```python
from build123d import *

# Parameters (mm, degrees)
F1_R      = 1
F2_DEPTH  = 2.2
F4_DEPTH  = 0.25
F6_DEPTH  = 2.2
F9_DEPTH  = 30
F11_DEPTH = 6.4
F13_R     = 2
F13_R_2   = 1
F14_DEPTH = 1


# Not quite as in the source:
# - a feature names something its author has since deleted; it is built from what else it names


with BuildPart() as f2:
    # F1 (on Front) → F2 (new body)
    with BuildSketch(Plane.XZ):
        with BuildLine():
            Line((7.35, 2), (7.35, 8.5))
            Line((7.35, 8.5), (0, 8.5))
            ThreePointArc((0, 8.5), (-2.1213203436, 7.6213203436), (-3, 5.5))
            Line((-3, 5.5), (-3, 5))
            ThreePointArc((-3, 5), (-2.8977774789, 4.2235428647), (-2.5980762114, 3.5))
            Line((-2.5980762114, 3.5), (-0.5775284417, 0.0003086038))
            Line((-0.5775284417, 0.0003086038), (0, -1))
            Line((0, -1), (0, 0))
            Line((0, 0), (2, 0))
            Line((2, 0), (7.35, 0))
            Line((7.35, 0), (7.35, 2))
        make_face()
        with Locations((0, 5)):
            Circle(F1_R, mode=Mode.SUBTRACT)
    extrude(amount=-F2_DEPTH)

    # F3 (on Front) → F4 (join)
    with BuildSketch(Plane.XZ):
        Polygon((7.35, 8.5), (4, 8.5), (4, 2), (4, 0), (7.35, 0), (7.35, 2), align=None)
    extrude(amount=F4_DEPTH)

    # F5 (on face) → F6 (join)
    with BuildSketch(Plane.XZ.offset(0.25)):
        with BuildLine():
            ThreePointArc((13.9434358481, 3.491991213), (14.2465762155, 4.2190734812), (14.35, 5))
            Line((14.35, 5), (14.35, 5.5))
            ThreePointArc((14.35, 5.5), (13.4713203436, 7.6213203436), (11.35, 8.5))
            Line((11.35, 8.5), (4, 8.5))
            Line((4, 8.5), (4, 2))
            Line((4, 2), (4, 0))
            Line((4, 0), (7.3888939805, 0))
            Line((7.3888939805, 0), (10.75, -1))
            Line((10.75, -1), (10.75, -2))
            Line((10.75, -2), (13.9434358481, 3.491991213))
        make_face()
        with BuildLine():
            Line((11.35, 3.5), (9.85, 3.5))
            ThreePointArc((9.85, 3.5), (8.35, 5), (9.85, 6.5))
            Line((9.85, 6.5), (11.35, 6.5))
            ThreePointArc((11.35, 6.5), (12.85, 5), (11.35, 3.5))
        make_face(mode=Mode.SUBTRACT)
    extrude(amount=F6_DEPTH)

    # F8 (on offset) → F9 (join)
    with BuildSketch(Plane.XZ.offset(6.45)):
        with BuildLine():
            Line((10.75, -2), (10.75, -1))
            Line((10.75, -1), (10.75, -0.9))
            ThreePointArc((10.75, -0.9), (10.4863961031, -0.2636038969), (9.85, 0))
            Line((9.85, 0), (7.3888939805, 0))
            Line((7.3888939805, 0), (7.3888939805, 0.6))
            ThreePointArc((7.3888939805, 0.6), (7.1252900836, 1.2363961031), (6.4888939805, 1.5))
            Line((6.4888939805, 1.5), (0.9, 1.5))
            ThreePointArc((0.9, 1.5), (0.2636038969, 1.2363961031), (0, 0.6))
            Line((0, 0.6), (0, -1))
            Line((0, -1), (0.5773502692, -2))
            Line((0.5773502692, -2), (2.6773502692, -2))
            Line((2.6773502692, -2), (2.6773502692, -1))
            Line((2.6773502692, -1), (4.6136751346, -1))
            Line((4.6136751346, -1), (4.6136751346, -2))
            Line((4.6136751346, -2), (6.7136751346, -2))
            Line((6.7136751346, -2), (6.7136751346, -1))
            Line((6.7136751346, -1), (8.65, -1))
            Line((8.65, -1), (8.65, -2))
            Line((8.65, -2), (10.75, -2))
        make_face()
    extrude(amount=-F9_DEPTH)

    # F10 (on offset) → F11 (cut)
    with BuildSketch(Plane.XZ.offset(6.45)):
        with BuildLine():
            ThreePointArc((0.9, 1.5), (0.2636038969, 1.2363961031), (0, 0.6))
            Line((0, 0.6), (0, -1))
            Line((0, -1), (0.5773502692, -2))
            Line((0.5773502692, -2), (2.0773502692, -2))
            Line((2.0773502692, -2), (2.0773502692, -0.8))
            Line((2.0773502692, -0.8), (3.6773515204, 1.5))
            Line((3.6773515204, 1.5), (0.9, 1.5))
        make_face()
    extrude(amount=-F11_DEPTH, mode=Mode.SUBTRACT)

    # F12: F2 across plane


with BuildPart() as f2_1:
    add(f2.part)
    add(f2.part.mirror(Plane(origin=(8.5554041441, -6.45, 4.0498921838), x_dir=(1, 0, 0), z_dir=(0, -1, 0))))

    # F13 (on face) → F14 (cut)
    with BuildSketch(Plane.XZ.offset(15.1)):
        with Locations((0, 5)):
            Circle(F13_R)
        with Locations((0, 5)):
            Circle(F13_R_2, mode=Mode.SUBTRACT)
    extrude(amount=-F14_DEPTH, mode=Mode.SUBTRACT)


solid = f2_1.part
```
Design review of the part built by this model. Coordinates are the model's own, in mm. A direction names the side the tool comes from. Round coordinates to 2 decimals unless told otherwise and drop trailing zeros. Write each loop counter-clockwise with the first axis right and the second up, starting at its lowest first coordinate (ties: lowest second). Pieces come first, ordered by that corner, then holes.
Item 1: The part is to be moulded in two halves that separate along Z. For faces 5 (the flat face through (11, -12, 6.5)), 6 (the flat face through (10.75, -6.4, -1.5)), 7 (the cylindrical face through (-2.1, -13.98, 7.64)), 8 (the flat face through (11, -1, 6.5)), say which applies: +Z half, -Z half, draft (parallel to the pull), parting line (faces both ways), or undercut.
Item 2: Clearance check with flat-ended pins moving along their axes: pin 1 Ø4.5 at (x, z) = (-1, 5.5) entering from -Y; pin 2 Ø0.5 at (y, z) = (-7.5, 0.5) entering from +X; pin 3 Ø1.2 at (y, z) = (-4.5, -1.5) entering from +X. State where each tip first meets the part, or that it passes through.
Item 3: We need section C-C on z = 2.25. Write out the cut boundary in (x, y).
Item 4: We need section D-D on x = 12. Write out the cut boundary in (y, z), and give its area (3 significant figures).
Item 5: We need section A-A on y = 18. Write out the cut boundary in (x, z), and give its area (3 significant figures).
Item 6: For faces 1 (the flat face through (11, -12.65, 3)), 2 (the flat face through (0, -26, 0)), 3 (the flat face through (9, -6, 0)), 4 (the flat face through (4, -1, 5)), list the 3-axis set-ups (+Z, -Z, +X, -X, +Y, -Y) from which the entire face can be reached by the end or side of a thin tool; tool diameter is ignored.
Item 7: We need section B-B on x = 5.75. Write out the cut boundary in (y, z).
Item 8: For probe 1 along Z at (x, y) = (0, -13.5); probe 2 along Y at (x, z) = (4.5, 4.5); probe 3 along Y at (x, z) = (-1.75, 7.25), list the stretches that pass through material, from the lowest coordinate up.
Returned:
1. face 5: undercut
1. face 6: draft
1. face 7: +Z half
1. face 8: undercut
2. pin 1: stops at y = -15.1
2. pin 2: stops at x = 7.39
2. pin 3: stops at x = 10.75
3. outline: (-1.88, -15.1) - (7.35, -15.1) - (7.35, -12.65) - (13.22, -12.65) - (13.22, -10.45) - (4, -10.45) - (4, -12.9) - (-1.88, -12.9) - close; (-1.88, 0) - (4, 0) - (4, -2.45) - (13.22, -2.45) - (13.22, -0.25) - (7.35, -0.25) - (7.35, 2.2) - (-1.88, 2.2) - close
4. outline: (-12.65, 0.15) - (-10.45, 0.15) - (-10.45, 3.65) - (-12.65, 3.65) - close; (-12.65, 6.35) - (-10.45, 6.35) - (-10.45, 8.43) - (-12.65, 8.43) - close; (-2.45, 0.15) - (-0.25, 0.15) - (-0.25, 3.65) - (-2.45, 3.65) - close; (-2.45, 6.35) - (-0.25, 6.35) - (-0.25, 8.43) - (-2.45, 8.43) - close
4. area: 24.5 mm2
5. outline: (0, -1) - (0.58, -2) - (2.68, -2) - (2.68, -1) - (4.61, -1) - (4.61, -2) - (6.71, -2) - (6.71, -1) - (8.65, -1) - (8.65, -2) - (10.75, -2) - (10.75, -0.9) arc R0.9 ccw to (9.85, 0) - (7.39, 0) - (7.39, 0.6) arc R0.9 ccw to (6.49, 1.5) - (0.9, 1.5) arc R0.9 ccw to (0, 0.6) - close
5. area: 27.9 mm2
6. face 1: +Z, +X, -Y
6. face 2: +Z, -Z, -X, -Y
6. face 3: +Z, +X
6. face 4: +Z, -X
7. outline: (-36.45, -2) - (23.55, -2) - (23.55, 1.5) - (2.2, 1.5) - (2.2, 8.5) - (-2.45, 8.5) - (-2.45, 1.5) - (-10.45, 1.5) - (-10.45, 8.5) - (-15.1, 8.5) - (-15.1, 1.5) - (-36.45, 1.5) - close
8. probe 1: z = -1 to 4, 6 to 8.5
8. probe 2: y = -15.1 to -10.45, -2.45 to 2.2
8. probe 3: y = -15.1 to -12.9, 0 to 2.2
